Design review of the part built by this model. Coordinates are the model's own, in mm. Coordinates: 2 decimals unless noted, no trailing zeros. Write each loop counter-clockwise with the first axis right and the second up, starting at its lowest first coordinate (ties: lowest second). Pieces come first, ordered by that corner, then holes.
Q1. For probe 1 along Z at (x, y) = (0.25, -2.25); probe 2 along X at (y, z) = (-0.5, 2.6); probe 3 along Z at (x, y) = (-1.75, 2.25), list the stretches that pass through material, from the lowest coordinate up.
Q2. Take a section at C-C (z = 3.9). Give the boundary of the cut face in (x, y), and give its area (3 significant figures).
Q3. Mouldability with a two-part tool opening along X and no side actions: class faces 1 (the flat face through (1.577, -2.756, 0.821)), 2 (the cylindrical face through (-0.631, 2.003, 3.415)), 3 (the flat face through (-2.744, 1.598, 0.821)), 4 (the cylindrical face through (0.748, 0.976, 2.416)) as pulls with the +X half, pulls with the -X half, needs draft (parallel to the pull), parting line crosses it, or undercut.
Q4. Insertion check: pin 1 (1.5 mm diameter, centred on x = 2.5, z = 2.5, fed in from +Y); pin 2 (1.5 mm diameter, centred on y = -2, z = 2, fed in from +X); pin 3 (1.9 mm diameter, centred on x = -1, y = 0, fed in from +Z); pin 4 (1 mm diameter, centred on y = -1, z = 2.5, fed in from +X). Each pin has a flat end and moves straight along its axis. Give the tip position at first contact, or say it passes through.
Autodesk Inventor part; units mm, degrees
ref_plane "YZ Plane" through (0, 0, 0) normal (1, 0, 0) x (0, 1, 0)
ref_plane "XZ Plane" through (0, 0, 0) normal (0, 1, 0) x (-1, 0, 0)
ref_plane "XY Plane" through (0, 0, 0) normal (0, 0, 1) x (1, 0, 0)
sketch "Sketch1" plane through (0, 0, 0) normal (1, 0, 0) x (0, 1, 0)
  line L0 (0, 0) -> (2.695, 0)
  line L1 (2.695, 0) -> (2.695, 0.1833)
  line L2 (2.695, 0.1833) -> (2.5117, 0.3667)
  line L3 (2.5117, 0.3667) -> (2.5117, 0.55)
  line L4 (2.5117, 0.55) -> (4.7625, 0.55)
  line L5 (4.7625, 0.55) -> (4.7625, 1.1)
  line L6 (4.7625, 1.1) -> (2.1, 1.1)
  line L7 (2.1, 1.1) -> (2.1, 1.2)
  arc A0 (2.1, 1.3908) -> (2.1, 1.2) centre (2.13, 1.2954) ccw
  line L8 (2.1, 1.6816) -> (2.1, 5.1)
  line L9 (2.1, 5.1) -> (0, 5.1)
  line L10 (0, 5.1) -> (0, 0)
  arc A1 (2.1, 1.6816) -> (2.1, 1.4908) centre (2.13, 1.5862) ccw
  line L11 (2.1, 1.3908) -> (2.1, 1.4908)
  dimension "d0" = 5.39
  dimension "d1" = 1.1
  dimension "d2" = 4.2
  dimension "d3" = 9.525
  dimension "d4" = 4
  dimension "d5" = 0.1
  dimension "d6" = 0.55
  dimension "d7" = 0.1833
  dimension "d8" = 0.1833
  dimension "d9" = 0.1833
  dimension "d10" = 0.03
  dimension "d11" = 0.1
  dimension "d12" = 0.1
revolve "Revolution1" add sketch "Sketch1" angle 360 about axis through (0, 0, 5.1) along (0, 0, -1)
sketch "Sketch2" plane through (0, 0, 0.55) normal (0, 0, -1) x (-1, 0, 0)
  line L0 (0.8507, 3.175) -> (2.3243, 2.3243)
  line L1 (2.3243, 2.3243) -> (3.175, 0.8507)
  line L2 (3.175, 0.8507) -> (3.175, -0.8507)
  line L3 (3.175, -0.8507) -> (2.3243, -2.3243)
  line L4 (2.3243, -2.3243) -> (0.8507, -3.175)
  line L5 (0.8507, -3.175) -> (-0.8507, -3.175)
  line L6 (-0.8507, -3.175) -> (-2.3243, -2.3243)
  line L7 (-2.3243, -2.3243) -> (-3.175, -0.8507)
  line L8 (-3.175, -0.8507) -> (-3.175, 0.8507)
  line L9 (-3.175, 0.8507) -> (-2.3243, 2.3243)
  line L10 (-2.3243, 2.3243) -> (-0.8507, 3.175)
  line L11 (-0.8507, 3.175) -> (0.8507, 3.175)
  circle A0 centre (0, 0) radius 4.7625
  dimension "d16" = 6.35
extrude "Extrusion1" cut sketch "Sketch2" against normal through all
hole "Hole1" at (0, 0, 5.1) direction (0, 0, -1) diameter 2.459 end through all countersink diameter 3.15 countersink angle 120
hole "Hole2" [suppressed]
equation "\"d0\" = C_"
equation "\"d1\" = A_"
equation "\"d2\" = B"
equation "\"d3\" = 1.5 * H_"
equation "\"d4\" = Length_Code"
equation "\"d5\" = Mark_1"
equation "\"d6\" = 0.5 * A_"
equation "\"d7\" = 0.166667 * A_"
equation "\"d8\" = 0.166667 * A_"
equation "\"d9\" = 0.166667 * A_"
equation "\"d10\" = Mark_2"
equation "\"d11\" = Mark_1"
equation "\"d12\" = Mark_1"
equation "\"d13\" = T_"
equation "\"d14\" = 1.05 * Thread"
equation "\"d53\" = Length_Code"
equation "\"d18\" = 1.05 * Thread"
equation "\"d20\" = T_"
equation "\"d16\" = H_"
equation "\"Length_Code\" = 4"
equation "\"T_\" = 4"
equation "\"A_\" = 1.1"
equation "\"B\" = 4.2"
equation "\"C_\" = 5.39"
equation "\"H_\" = 6.35"
equation "\"Mark_1\" = 0.1"
equation "\"Mark_2\" = 0.03"
equation "\"Thread\" = 3"
equation "\"Min_Thick\" = 1.6"
equation "\"B_Hole\" = 5.41"
equation "\"Min_Depht\" = 1.1"
equation "\"Min_Dist\" = 4.8"
properties part number "CSS-M3-4" material "Stainless Steel"
Response:
1. probe 1: z = 0 to 1.1
1. probe 2: x = -2.04 to -1.12, 1.12 to 2.04
1. probe 3: z = 0.55 to 1.1
2. outline: circle Ø4.2 at (0, 0); hole circle Ø2.46 at (0, 0)
2. area: 9.11 mm2
3. face 1: pulls with the +X half
3. face 2: parting line crosses it
3. face 3: pulls with the -X half
3. face 4: undercut
4. pin 1: stops at y = 1.16
4. pin 2: stops at x = 1.69
4. pin 3: stops at z = 5.1
4. pin 4: stops at x = 2.04
